The model under review builds one solid part; all positions refer to its coordinate system, in mm. Coordinates: 2 decimals unless noted, no trailing zeros.
```python
from build123d import *

# Parameters (mm, degrees)
CROQUIS1_W              = 230
CROQUIS1_H              = 230
SALIENTE_EXTRUIR2_DEPTH = 3
REDONDEO1_R             = 30
REDONDEO2_R             = 30
REDONDEO3_R             = 30
REDONDEO4_R             = 30
CROQUIS2_R              = 1.5
CROQUIS2_R_2            = 15
CROQUIS2_R_3            = 1.6
CROQUIS2_W              = 5
CROQUIS2_H              = 5
CROQUIS2_W_2            = 4
CROQUIS2_H_2            = 4
CROQUIS2_W_3            = 6.425619835
CORTAR_EXTRUIR2_DEPTH   = 3


with BuildPart() as part:
    # Croquis1 → Saliente-Extruir2 (new body)
    with BuildSketch(Plane.XY):
        Rectangle(CROQUIS1_W, CROQUIS1_H)
    extrude(amount=SALIENTE_EXTRUIR2_DEPTH)

    # Redondeo1
    redondeo1_edges = [part.edges().sort_by_distance(p)[0] for p in [
        (-115, 115, 1.5),
    ]]
    fillet(redondeo1_edges, radius=REDONDEO1_R)

    # Redondeo2
    redondeo2_edges = [part.edges().sort_by_distance(p)[0] for p in [
        (-115, -115, 1.5),
    ]]
    fillet(redondeo2_edges, radius=REDONDEO2_R)

    # Redondeo3
    redondeo3_edges = [part.edges().sort_by_distance(p)[0] for p in [
        (115, -115, 1.5),
    ]]
    fillet(redondeo3_edges, radius=REDONDEO3_R)

    # Redondeo4
    redondeo4_edges = [part.edges().sort_by_distance(p)[0] for p in [
        (115, 115, 1.5),
    ]]
    fillet(redondeo4_edges, radius=REDONDEO4_R)

    # Croquis2 → Cortar-Extruir2 (cut)
    with BuildSketch(Plane.XY.offset(3)):
        with Locations((-22.88, 46.75)):
            Circle(CROQUIS2_R)
        with Locations((-70.13, 46.75)):
            Circle(CROQUIS2_R)
        with Locations((-70.13, 69.25)):
            Circle(CROQUIS2_R)
        with Locations((-22.88, 69.25)):
            Circle(CROQUIS2_R)
        with Locations((22.88, 69.25)):
            Circle(CROQUIS2_R)
        with Locations((22.88, 46.75)):
            Circle(CROQUIS2_R)
        with Locations((70.13, 46.75)):
            Circle(CROQUIS2_R)
        with Locations((70.13, 69.25)):
            Circle(CROQUIS2_R)
        with Locations((70.13, -69.25)):
            Circle(CROQUIS2_R)
        with Locations((70.13, -46.75)):
            Circle(CROQUIS2_R)
        with Locations((22.88, -69.25)):
            Circle(CROQUIS2_R)
        with Locations((22.88, -46.75)):
            Circle(CROQUIS2_R)
        with Locations((-22.88, -46.75)):
            Circle(CROQUIS2_R)
        with Locations((-22.88, -69.25)):
            Circle(CROQUIS2_R)
        with Locations((-70.13, -69.25)):
            Circle(CROQUIS2_R)
        with Locations((-70.13, -46.75)):
            Circle(CROQUIS2_R)
        Circle(CROQUIS2_R_2)
        with Locations((42.973295778, -34.981331753)):
            Circle(CROQUIS2_R)
        with Locations((-99.142135624, 99.142135624)):
            Circle(CROQUIS2_R)
        with Locations((99.142135624, 99.142135624)):
            Circle(CROQUIS2_R)
        with Locations((99.142135624, -99.142135624)):
            Circle(CROQUIS2_R)
        with Locations((-99.142135624, -99.142135624)):
            Circle(CROQUIS2_R)
        with Locations((-49, 15)):
            Circle(CROQUIS2_R_3)
        with Locations((-49, -15)):
            Circle(CROQUIS2_R_3)
        with Locations((49, 15)):
            Circle(CROQUIS2_R_3)
        with Locations((49, -15)):
            Circle(CROQUIS2_R_3)
        with Locations((15, 84)):
            Circle(CROQUIS2_R_3)
        with Locations((-15, 84)):
            Circle(CROQUIS2_R_3)
        with Locations((-102.407537284, 38.45)):
            Circle(CROQUIS2_R)
        with Locations((-65.507537284, 38.45)):
            Circle(CROQUIS2_R)
        with Locations((-65.507537284, 1.55)):
            Circle(CROQUIS2_R)
        with Locations((-102.407537284, 1.55)):
            Circle(CROQUIS2_R)
        with Locations((102.407537284, 1.55)):
            Circle(CROQUIS2_R)
        with Locations((65.507537284, 1.55)):
            Circle(CROQUIS2_R)
        with Locations((65.507537284, 38.45)):
            Circle(CROQUIS2_R)
        with Locations((102.407537284, 38.45)):
            Circle(CROQUIS2_R)
        with Locations((-90, -90)):
            Circle(CROQUIS2_R)
        with Locations((90, -90)):
            Circle(CROQUIS2_R)
        with Locations((90, -25)):
            Circle(CROQUIS2_R)
        with Locations((-90, -25)):
            Circle(CROQUIS2_R)
        with Locations((39.09562129, 86.314599105)):
            Circle(CROQUIS2_R)
        with Locations((65.507537284, 106.866636631)):
            Circle(CROQUIS2_R)
        with Locations((-6.05453105, 58.000440639)):
            Rectangle(CROQUIS2_W, CROQUIS2_H)
        with Locations((6.05453105, 58.000440639)):
            Rectangle(CROQUIS2_W, CROQUIS2_H)
        with Locations((6.05453105, -58.000440639)):
            Rectangle(CROQUIS2_W, CROQUIS2_H)
        with Locations((-6.05453105, -58.000440639)):
            Rectangle(CROQUIS2_W, CROQUIS2_H)
        with Locations((35.684074381, 0)):
            Rectangle(CROQUIS2_W_2, CROQUIS2_H_2)
        with Locations((0, 72.426144441)):
            Rectangle(CROQUIS2_W_2, CROQUIS2_H_2)
        with Locations((-35.684074381, 0)):
            Rectangle(CROQUIS2_W_2, CROQUIS2_H_2)
        with Locations((52.672582405, 96.879308397)):
            Rectangle(CROQUIS2_W_3, CROQUIS2_H)
    extrude(amount=-CORTAR_EXTRUIR2_DEPTH, mode=Mode.SUBTRACT)


solid = part.part
```
(1) Wall thickness on probe 1 along Y at (x, z) = (70.13, 0.6); probe 2 along X at (y, z) = (57.5, 1.8); probe 3 along Y at (x, z) = (49, 1.4): over which ranges is each line inside the solid? List them lowest first.
A:
probe 1: y = -115 to -70.75, -67.75 to -48.25, -45.25 to 45.25, 48.25 to 67.75, 70.75 to 115
probe 2: x = -115 to -8.55, -3.55 to 3.55, 8.55 to 115
probe 3: y = -115 to -16.6, -13.4 to 13.4, 16.6 to 115
(2) For pin 1 Ø1 at (x, z) = (-86, 2) entering from -Y; pin 2 Ø1.8 at (x, y) = (-22.88, 46.75) entering from +Z, all flat-tipped, find the tip position at first contact; note any pin that passes through.
A:
pin 1: stops at y = -115
pin 2: passes through
(3) We need section A-A, the plane z = 1. Count the separate pieces of the cut face and the enclosed holes in it, and give its area (3 significant figures).
A:
separate pieces: 1
enclosed holes: 50
area: 50,900 mm2
(4) Draft analysis for pull direction Y (two halves, no side actions). For faces 1 (the face through (-14.985, 0.66, 1.521)), 2 (the face through (-106.445, 105.979, 1.521)), 3 (the face through (24, 2, 0)), 4 (the face through (-106.445, -105.979, 1.521)), state which applies: released by +Y, released by -Y, zero draft, split by the parting line, or undercut.
A:
face 1: undercut
face 2: released by +Y
face 3: zero draft
face 4: released by -Y
